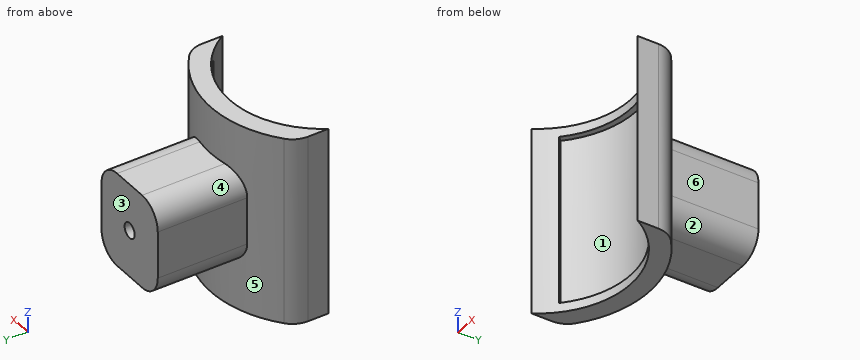
from build123d import *

# Parameters (mm, degrees)
F1_DEPTH      = 40
F3_W          = 18
F3_H          = 20
F4_DEPTH      = 10
F4_DEPTH_BACK = 10
F7_DEPTH      = 36
F8_R          = 1.625
F9_DEPTH      = 15
F10_R         = 5


with BuildPart() as f1:
    # F0 (on Top) → F1 (new body)
    with BuildSketch(Plane.XY):
        with BuildLine():
            ThreePointArc((-17, 0), (0, 9.697015), (17, 0))
            Line((17, 0), (17, 4.354045))
            ThreePointArc((17, 4.354045), (16.527693, 6.475365), (15.2, 8.195919))
            ThreePointArc((15.2, 8.195919), (0, 13.697015), (-15.2, 8.195919))
            ThreePointArc((-15.2, 8.195919), (-16.527693, 6.475365), (-17, 4.354045))
            Line((-17, 4.354045), (-17, 0))
        make_face()
    extrude(amount=F1_DEPTH)

    # F3 (on offset) → F4 (join, two sides)
    with BuildSketch(Plane.XY.offset(20)) as f4_sk:
        with Locations((0, 20.889152)):
            Rectangle(F3_W, F3_H)
    extrude(amount=F4_DEPTH)
    extrude(f4_sk.sketch, amount=-F4_DEPTH_BACK)

    # F6 (on offset) → F7 (cut)
    with BuildSketch(Plane.XY.offset(2)):
        with BuildLine():
            Line((14, 3.877647), (14.886076, 4.759333))
            ThreePointArc((14.886076, 4.759333), (0, 10.947015), (-14.886076, 4.759333))
            Line((-14.886076, 4.759333), (-14, 3.877647))
            ThreePointArc((-14, 3.877647), (0, 9.697015), (14, 3.877647))
        make_face()
    extrude(amount=F7_DEPTH, mode=Mode.SUBTRACT)

    # F8 (on face) → F9 (cut)
    with BuildSketch(Plane(origin=(0, 30.889152, 0), x_dir=(-1, 0, 0), z_dir=(0, 1, 0))):
        with Locations((0, 20)):
            Circle(F8_R)
    extrude(amount=-F9_DEPTH, mode=Mode.SUBTRACT)

    # F10
    f10_edges = [f1.edges().sort_by_distance(p)[0] for p in [
        (9, 21.407425, 30),
        (-9, 21.407425, 30),
        (-9, 21.407425, 10),
        (9, 21.407425, 10),
    ]]
    fillet(f10_edges, radius=F10_R)


solid = f1.part
The model under review builds one solid part; all positions refer to its coordinate system, in mm. Face numbers are marked on the shaded views. A direction names the side the tool comes from. Round coordinates to 2 decimals unless told otherwise and drop trailing zeros. Loops run counter-clockwise (first coordinate to the right, second up) from the corner with the lowest first, then second, coordinate; pieces in that order, holes last. Notation, with made-up numbers: (78.25, -17) -> (89.25, -17) arc R22 cw to (89.25, 10) -> close; hole circle Ø3 at (57, 30). An arc over 180 degrees is marked (long way). Return JSON: item names as keys, results as strings.
(1) Add section A-A on y = 17. Write out the cut boundary in (x, z) (3 decimals), plus the area to 3 significant figures.
Solved:
{"outline": "(-9, 15) arc R5 ccw to (-4, 10) -> (4, 10) arc R5 ccw to (9, 15) -> (9, 25) arc R5 ccw to (4, 30) -> (-4, 30) arc R5 ccw to (-9, 25) -> close; hole circle Ø3.25 at (0, 20)", "area": "330 mm2"}
(2) For the marked faces 4, 5 and 6, list the 3-axis set-ups (+Z, -Z, +X, -X, +Y, -Y) from which the entire face can be reached by the end or side of a thin tool; tool diameter is ignored.
Solved:
{"face 4": "+Z, -X, +Y", "face 5": "+Y", "face 6": "+Z, -Z, +X, +Y"}
(3) For pin 1 (1 mm diameter, centred on x = 0, z = 19.5, fed in from +Y); pin 2 (12 mm diameter, centred on x = -5.5, y = 20.5, fed in from -Z); pin 3 (12 mm diameter, centred on x = -0.5, y = 7, fed in from -Z); pin 4 (5 mm diameter, centred on y = 18.5, z = 20.5, fed in from -X), all flat-tipped, find the tip position at first contact; note any pin that passes through.
Solved:
{"pin 1": "y = 15.89", "pin 2": "z = 10", "pin 3": "z = 0", "pin 4": "x = -9"}
(4) The part is to be moulded in two halves that separate along Z. For the marked faces 1, 2 and 3, say which applies: released by +Z, released by -Z, zero draft, split by the parting line, or undercut.
Solved:
{"face 1": "undercut", "face 2": "released by -Z", "face 3": "zero draft"}
(5) Add section D-D on x = 13. Write out the cut boundary in (y, z).
Solved:
{"outline": "(4.82, 0) -> (9.82, 0) -> (9.82, 40) -> (4.82, 40) -> (4.82, 38) -> (6.44, 38) -> (6.44, 2) -> (4.82, 2) -> close"}
(6) Add section C-C on z = 27.5. Write out the cut boundary in (x, y).
Solved:
{"outline": "(-17, 0) arc R19.75 cw to (-14, 3.88) -> (-14.89, 4.76) arc R21 cw to (14.89, 4.76) -> (14, 3.88) arc R19.75 cw to (17, 0) -> (17, 4.35) arc R5 ccw to (15.2, 8.2) arc R23.75 ccw to (8.33, 12.19) -> (8.33, 30.89) -> (-8.33, 30.89) -> (-8.33, 12.19) arc R23.75 ccw to (-15.2, 8.2) arc R5 ccw to (-17, 4.35) -> close"}
(7) For line 1 (Z direction, x = 0, y = 27.25) (3 decimals); line 2 (Z direction, x = -3, y = 10); line 3 (X direction, y = 8, z = 25), list the stretches that pass through material, from the lowest coordinate up.
Solved:
{"line 1": "10 to 18.375, 21.625 to 30", "line 2": "0 to 2, 38 to 40", "line 3": "-15.42 to -10.73, 10.73 to 15.42"}
(8) Add section B-B on x = 0. Write out the cut boundary in (y, z) (3 decimals).
Solved:
{"outline": "(9.697, 0) -> (13.697, 0) -> (13.697, 10) -> (30.889, 10) -> (30.889, 18.375) -> (15.889, 18.375) -> (15.889, 21.625) -> (30.889, 21.625) -> (30.889, 30) -> (13.697, 30) -> (13.697, 40) -> (9.697, 40) -> (9.697, 38) -> (10.947, 38) -> (10.947, 2) -> (9.697, 2) -> close"}
